Geometry: final body of the model. Coordinates: model frame, mm. Face numbers are marked on the shaded views. A direction names the side the tool comes from. Give positions to 0.01 mm unless a question says otherwise; leave off trailing zeros. Write each loop counter-clockwise with the first axis right and the second up, starting at its lowest first coordinate (ties: lowest second). Pieces come first, ordered by that corner, then holes. Notation, with made-up numbers: M 47,-32 L 80,-32 A15 ccw 80,-26 Z; hole C -14,31 d1. An arc over 180 degrees is marked long. Answer as a JSON object with one key per item and string values.
from build123d import *

# Parameters (mm, degrees)
SKETCH1_R                  = 6.35
BOSS_EXTRUDE1_DEPTH        = 5
SKETCH2_R                  = 7
BOSS_EXTRUDE2_DEPTH        = 2
BOSS_EXTRUDE3_START        = -7
SKETCH2_2_R                = 7
BOSS_EXTRUDE3_DEPTH        = 2
CHAMFER1_SIZE              = 1
SKETCH3_W                  = 8.3
SKETCH3_H                  = 6.3
CUT_EXTRUDE1_DEPTH         = 14.37908816
BOSS_EXTRUDE4_DEPTH        = 1
BOSS_EXTRUDE4_DEPTH_BACK   = 1
SKETCH6_R                  = 2.5
SKETCH6_R_2                = 1.1
BOSS_EXTRUDE4_2_DEPTH      = 1
BOSS_EXTRUDE4_2_DEPTH_BACK = 1
BOSS_EXTRUDE4_3_DEPTH      = 1
BOSS_EXTRUDE4_3_DEPTH_BACK = 1
BOSS_EXTRUDE4_4_DEPTH      = 1
BOSS_EXTRUDE4_4_DEPTH_BACK = 1
SKETCH7_W                  = 8.3
SKETCH7_H                  = 6.3
BOSS_EXTRUDE5_DEPTH        = 2


with BuildPart() as part:
    # Sketch1 → Boss-Extrude1 (new body)
    with BuildSketch(Plane(origin=(0, 0, 0), x_dir=(1, 0, 0), z_dir=(0, 1, 0))):
        with Locations(Location((0, 0, 0), (0, 0, 270))):
            Circle(SKETCH1_R)
    extrude(amount=-BOSS_EXTRUDE1_DEPTH)

    # Sketch2 → Boss-Extrude2 (add)
    with BuildSketch(Plane(origin=(0, 0, 0), x_dir=(1, 0, 0), z_dir=(0, 1, 0))):
        with Locations(Location((0, 0, 0), (0, 0, 270))):
            Circle(SKETCH2_R)
    extrude(amount=BOSS_EXTRUDE2_DEPTH)

    # Sketch2<2> → Boss-Extrude3 (add)
    with BuildSketch(Plane(origin=(0, 0, 0), x_dir=(1, 0, 0), z_dir=(0, 1, 0)).offset(BOSS_EXTRUDE3_START)):
        with Locations(Location((0, 0, 0), (0, 0, 270))):
            Circle(SKETCH2_2_R)
    extrude(amount=BOSS_EXTRUDE3_DEPTH)

    # Chamfer1
    # the kernel refuses this chamfer: 1 mm, written as the material it takes off along each edge
    with BuildSketch(Plane(origin=(0, 0, 0), x_dir=(0, 0, 1), z_dir=(-1, 0, 0))) as chamfer1_piece_1_section:
        Polygon((7 - CHAMFER1_SIZE, 0), (7, CHAMFER1_SIZE), (7, 0), align=None)
    chamfer1_piece_1 = revolve(axis=Axis((0, 0, 0), (0, 1, 0)), mode=Mode.PRIVATE)
    chamfer1_piece_1 = chamfer1_piece_1 - Plane(origin=(0, 0.669896582, 0), x_dir=(0, 0, 1), z_dir=(0, 1, 0)) * Cylinder(6.35, 28, mode=Mode.PRIVATE)
    add(chamfer1_piece_1, mode=Mode.SUBTRACT)
    with BuildSketch(Plane(origin=(0, -7, 0), x_dir=(0, 0, 1), z_dir=(-1, 0, 0))) as chamfer1_piece_2:
        Polygon((7, CHAMFER1_SIZE), (7 - CHAMFER1_SIZE, 0), (7, 0), align=None)
    revolve(axis=Axis((0, -7, 0), (0, 1, 0)), mode=Mode.SUBTRACT)

    # Sketch3 → Cut-Extrude1 (cut, through all)
    with BuildSketch(Plane.XZ.offset(7)):
        Rectangle(SKETCH3_W, SKETCH3_H)
    extrude(amount=-CUT_EXTRUDE1_DEPTH, mode=Mode.SUBTRACT)



with BuildPart() as body_2:
    # Sketch6 → Boss-Extrude4 (new, two sides: drawn at the far end of the back side and taken through both)
    with BuildSketch(Plane(origin=(0, 2, 0), x_dir=(1, 0, 0), z_dir=(0, 1, 0)).offset(-BOSS_EXTRUDE4_DEPTH_BACK)):
        with Locations(Location((-18, -11, 0), (0, 0, 270))):
            Circle(SKETCH6_R)
        with Locations(Location((-18, -11, 0), (0, 0, 270))):
            Circle(SKETCH6_R_2, mode=Mode.SUBTRACT)
    extrude(amount=BOSS_EXTRUDE4_DEPTH + BOSS_EXTRUDE4_DEPTH_BACK)


with BuildPart() as body_3:
    # Sketch6 → Boss-Extrude4 2 (new, two sides: drawn at the far end of the back side and taken through both)
    with BuildSketch(Plane(origin=(0, 2, 0), x_dir=(1, 0, 0), z_dir=(0, 1, 0)).offset(-BOSS_EXTRUDE4_2_DEPTH_BACK)):
        with Locations(Location((18, -11, 0), (0, 0, 270))):
            Circle(SKETCH6_R)
        with Locations(Location((18, -11, 0), (0, 0, 270))):
            Circle(SKETCH6_R_2, mode=Mode.SUBTRACT)
    extrude(amount=BOSS_EXTRUDE4_2_DEPTH + BOSS_EXTRUDE4_2_DEPTH_BACK)


with BuildPart() as body_4:
    # Sketch6 → Boss-Extrude4 3 (new, two sides: drawn at the far end of the back side and taken through both)
    with BuildSketch(Plane(origin=(0, 2, 0), x_dir=(1, 0, 0), z_dir=(0, 1, 0)).offset(-BOSS_EXTRUDE4_3_DEPTH_BACK)):
        with Locations(Location((18, 12, 0), (0, 0, 270))):
            Circle(SKETCH6_R)
        with Locations(Location((18, 12, 0), (0, 0, 270))):
            Circle(SKETCH6_R_2, mode=Mode.SUBTRACT)
    extrude(amount=BOSS_EXTRUDE4_3_DEPTH + BOSS_EXTRUDE4_3_DEPTH_BACK)


with BuildPart() as body_5:
    # Sketch6 → Boss-Extrude4 4 (new, two sides: drawn at the far end of the back side and taken through both)
    with BuildSketch(Plane(origin=(0, 2, 0), x_dir=(1, 0, 0), z_dir=(0, 1, 0)).offset(-BOSS_EXTRUDE4_4_DEPTH_BACK)):
        with Locations(Location((-18, 12, 0), (0, 0, 270))):
            Circle(SKETCH6_R)
        with Locations(Location((-18, 12, 0), (0, 0, 270))):
            Circle(SKETCH6_R_2, mode=Mode.SUBTRACT)
    extrude(amount=BOSS_EXTRUDE4_4_DEPTH + BOSS_EXTRUDE4_4_DEPTH_BACK)


with BuildPart() as part_1:
    add(part.part)

    add(body_2.part)  # Boss-Extrude5 merges body 2

    add(body_3.part)  # Boss-Extrude5 merges body 3

    add(body_4.part)  # Boss-Extrude5 merges body 4

    add(body_5.part)  # Boss-Extrude5 merges body 5
    # Sketch7 → Boss-Extrude5 (add)
    with BuildSketch(Plane(origin=(0, 3, 0), x_dir=(1, 0, 0), z_dir=(0, 1, 0))):
        Polygon((-19.767766953, 10.232233047), (-16.232233047, 10.232233047), (-16.232233047, 13.767766953), (0, 7), (7, 7.572180743), (15.5, 12), (16.192434296, 10.272948691), (8.334514261, 4.869137674), (7, 0), (11.058001897, -11), (15.5, -11), (18, -13.5), (7.583003583, -13.5), (0, -7), (-16.232233047, -12.767766953), (-16.232233047, -9.232233047), (-19.767766953, -9.232233047), (-7, 0), align=None)
        Rectangle(SKETCH7_W, SKETCH7_H, mode=Mode.SUBTRACT)
    extrude(amount=-BOSS_EXTRUDE5_DEPTH)


solid = part_1.part
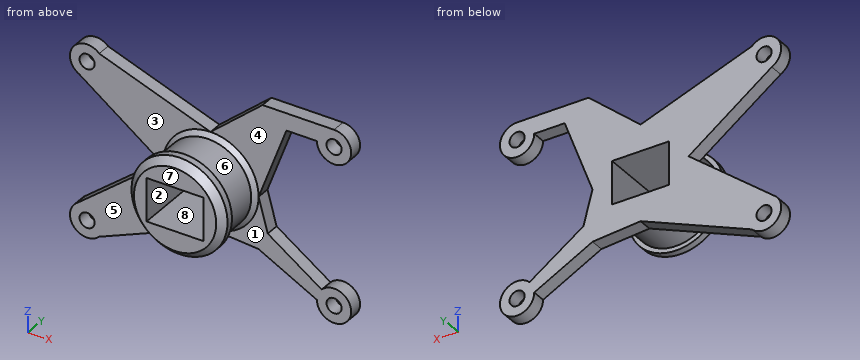
1) Cut plane A-A on x = -11. Return loops of the section in (y, z), and give its area (3 significant figures).
Geometry check:
{"outline": "M 1,-11.59 L 3,-11.59 L 3,-3.21 L 1,-3.21 Z; M 1,2.89 L 3,2.89 L 3,10.91 L 1,10.91 Z", "area": "32.8 mm2"}
2) Line query: line 1 (Y direction, x = -14, z = 11); line 2 (X direction, y = 0.5, z = -1); line 3 (Z direction, x = -14, y = 2). Output: solid intervals per line, ascending. Write a range as from..to.
Geometry check:
{"line 1": "y = 1..3", "line 2": "x = -6.42..-4.15, 4.15..6.42", "line 3": "z = -12.84..-5.61, 5.06..11.97"}
3) Contact query for flat-ended pins moving along their axis: P1, Ø2.5, axis at x = 18, z = -12, coming from the -Y side; P2, Ø5, axis at y = 1, z = 1, coming from the +X side; P3, Ø11.5, axis at x = 8, z = -9.5, coming from the -Y side. Output: stop coordinate, or through.
Geometry check:
{"P1": "stops at y = 1", "P2": "stops at x = 8.29", "P3": "stops at y = -6.33"}
4) Cut plane B-B on y = -2.75. Return loops of the section in (x, z).
Geometry check:
{"outline": "C 0,0 d12.7; hole M -4.15,-3.15 L 4.15,-3.15 L 4.15,3.15 L -4.15,3.15 Z"}
5) Pull-direction query (X, two-part tool) for the marked faces 6, 7 and 8; classes: pulls with the +X half, pulls with the -X half, needs draft (parallel to the pull), parting line crosses it, or undercut.
Geometry check:
{"face 6": "parting line crosses it", "face 7": "needs draft", "face 8": "undercut"}
6) Cut plane C-C on x = -18. Return loops of the section in (y, z).
Geometry check:
{"outline": "M 1,-14.5 L 3,-14.5 L 3,-13.1 L 1,-13.1 Z; M 1,-10.9 L 3,-10.9 L 3,-8.82 L 1,-8.82 Z; M 1,7.95 L 3,7.95 L 3,9.9 L 1,9.9 Z; M 1,12.1 L 3,12.1 L 3,13.5 L 1,13.5 Z"}
7) Set-up query: the marked faces 1, 2, 3, 4 and 5. Return all of +Z, -Z, +X, -X, +Y, -Y with unobstructed straight access to the full face (end or side cutting, diameter ignored); none if empty.
Geometry check:
{"face 1": "-Z, +X, -Y", "face 2": "+Y, -Y", "face 3": "+Z, -X, -Y", "face 4": "+Z, +X, -Y", "face 5": "-Z, -X, -Y"}
